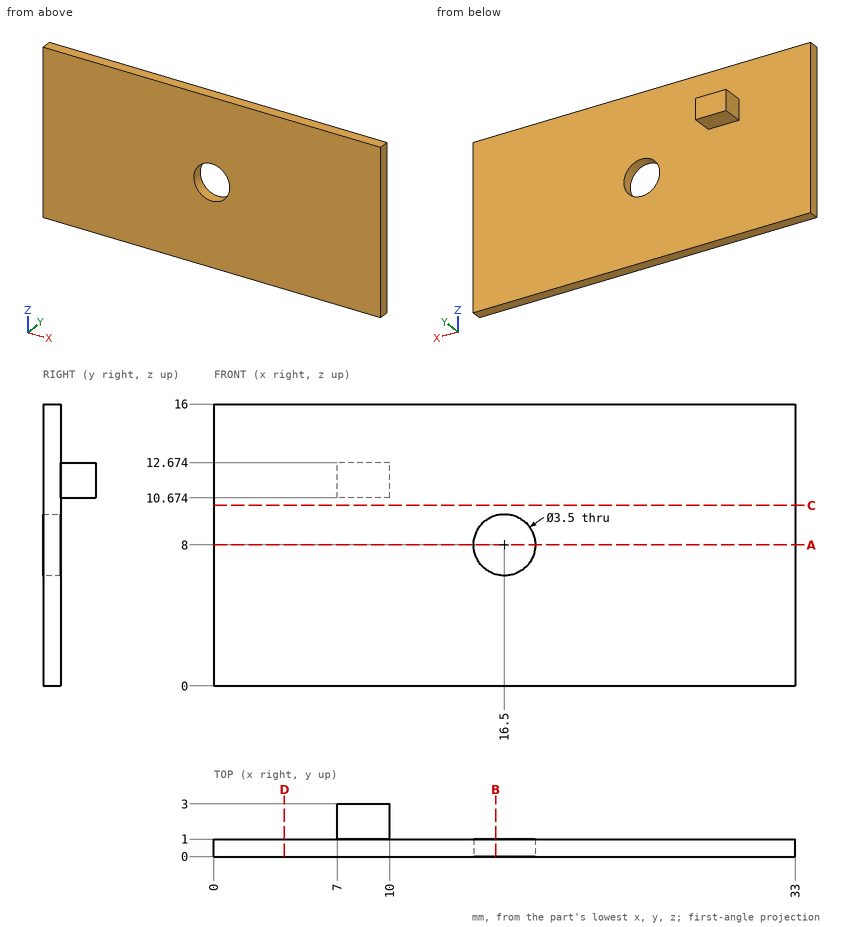
Geometry check sheet. Reference: drawing and pictorial views, mm from the part's lowest x, y, z. Give positions to 0.01 mm unless a question says otherwise; leave off trailing zeros. Order: outer loops, then holes, each group sorted by start corner. A loop starts at its lowest first (then second) coordinate and runs counter-clockwise, first axis right, second up. Notation, with made-up numbers: M 34,77.5 L 75,77.5 A22 cw 75,83.5 Z; hole C 9.5,26 d6. An arc over 180 degrees is marked long. Answer in a Markdown table with one row per item. Add a question column.
Q1. Sectioned sample at D-D, the plane x = 4. Record the boundary of the cut face in (y, z), and give its area (3 significant figures).
Q2. Sectioned sample at B-B, the plane x = 16. Record the boundary of the cut face in (y, z).
Q3. Sectioned sample at A-A, the plane z = 8. Record the boundary of the cut face in (x, y).
Q4. Thickness scan on L1, parallel to X at y = 0.5, z = 8; L2, parallel to Y at x = 17, z = 0.75; L3, parallel to Z at x = 17, y = 0.25. Record the ranges inside material, lowest first.
Q5. Sectioned sample at C-C, the plane z = 10.25. Record the boundary of the cut face in (x, y).
Q6. Gauge pin test, flat ends, axial feed: pin 1 Ø3 at (x, z) = (8, 2.5) entering from +Y; pin 2 Ø1 at (x, z) = (25.5, 5.5) entering from -Y; pin 3 Ø3 at (x, z) = (16.5, 8) entering from -Y; pin 4 Ø0.6 at (y, z) = (2, 12) entering from +X. Record the tip position at first contact, or that the pin passes through.
Verdict:
| question | item | result |
|---|---|---|
| 1 | outline | M 0,0 L 1,0 L 1,16 L 0,16 Z |
| 1 | area | 16.0 mm² |
| 2 | outline | M 0,0 L 1,0 L 1,6.32 L 0,6.32 Z; M 0,9.68 L 1,9.68 L 1,16 L 0,16 Z |
| 3 | outline | M 0,0 L 14.75,0 L 14.75,1 L 0,1 Z; M 18.25,0 L 33,0 L 33,1 L 18.25,1 Z |
| 4 | L1 | 0 to 14.75, 18.25 to 33 |
| 4 | L2 | 0 to 1 |
| 4 | L3 | 0 to 6.32, 9.68 to 16 |
| 5 | outline | M 0,0 L 33,0 L 33,1 L 0,1 Z |
| 6 | pin 1 | y = 1 |
| 6 | pin 2 | y = 0 |
| 6 | pin 3 | through |
| 6 | pin 4 | x = 10 |
